from build123d import *

# Parameters (mm, degrees)
BOSS_EXTRU_1_DEPTH      = 1.5
BOSS_EXTRU_2_DEPTH      = 13.5
D_GAGEMENT_M32_D        = 3.4
D_GAGEMENT_M32_DEPTH    = 10
D_GAGEMENT_M32_TIP      = 1.021463052
D_GAGEMENT_M31_D        = 3.4
D_GAGEMENT_M31_DEPTH    = 10
D_GAGEMENT_M31_TIP      = 1.021463052
ESQUISSE12_W            = 13.5
ESQUISSE12_H            = 13.5
ENL_V_MAT_EXTRU_1_DEPTH = 1.5
CONG_1_R                = 1
CONG_2_R                = 1
D_GAGEMENT_M33_D        = 3.4
D_GAGEMENT_M33_DEPTH    = 10
D_GAGEMENT_M33_TIP      = 1.021463052


# Some blends are built 0.0001 mm under size
with BuildPart() as part:
    # Esquisse2 → Boss.-Extru.1 (new body)
    with BuildSketch(Plane.XY.offset(1.5)):
        Polygon((-25.392437762, 124.305889048), (-178.410591433, 124.305889048), (-178.410591433, 149.305889048), (-222.374284091, 149.305889048), (-222.374284091, 124.305889048), (-375.392437762, 124.305889048), (-375.392437762, 109.305889048), (-207.374284091, 109.305889048), (-207.374284091, 134.305889048), (-193.410591433, 134.305889048), (-193.410591433, 109.305889048), (-25.392437762, 109.305889048), align=None)
    extrude(amount=BOSS_EXTRU_1_DEPTH)

    # Esquisse3 → Boss.-Extru.2 (add)
    with BuildSketch(Plane.XY.offset(3)):
        Polygon((-375.392437762, 122.805889048), (-220.874284091, 122.805889048), (-220.874284091, 147.805889048), (-179.910591433, 147.805889048), (-179.910591433, 122.805889048), (-25.392437762, 122.805889048), (-25.392437762, 124.305889048), (-178.410591433, 124.305889048), (-178.410591433, 149.305889048), (-222.374284091, 149.305889048), (-222.374284091, 124.305889048), (-375.392437762, 124.305889048), align=None)
    extrude(amount=BOSS_EXTRU_2_DEPTH)

    # Dégagement M32
    with Locations(Plane(origin=(-229.874284091, 116.805889048, 3), x_dir=(1, 0, 0), z_dir=(0, 0, 1))):
        with Locations((0, 0), (-70.518153671, 0), (-138.018153671, 0), (58.963692658, 0), (129.481846329, 0), (196.981846329, 0)):
            Hole(D_GAGEMENT_M32_D / 2, depth=D_GAGEMENT_M32_DEPTH)
            with Locations((0, 0, -(D_GAGEMENT_M32_DEPTH + D_GAGEMENT_M32_TIP / 2))):  # 118° drill point
                Cone(0, D_GAGEMENT_M32_D / 2, D_GAGEMENT_M32_TIP, mode=Mode.SUBTRACT)

    # Dégagement M31
    with Locations(Plane(origin=(-214.874284091, 137.305889048, 3), x_dir=(1, 0, 0), z_dir=(0, 0, 1))):
        with Locations((0, 0), (28.963692658, 0)):
            Hole(D_GAGEMENT_M31_D / 2, depth=D_GAGEMENT_M31_DEPTH)
            with Locations((0, 0, -(D_GAGEMENT_M31_DEPTH + D_GAGEMENT_M31_TIP / 2))):  # 118° drill point
                Cone(0, D_GAGEMENT_M31_D / 2, D_GAGEMENT_M31_TIP, mode=Mode.SUBTRACT)

    # Esquisse12 → Enlèv. mat.-Extru.1 (cut)
    with BuildSketch(Plane.XY.offset(3)):
        with Locations((-214.124284091, 116.055889048)):
            Rectangle(ESQUISSE12_W, ESQUISSE12_H)
        with Locations((-186.660591433, 116.055889048)):
            Rectangle(ESQUISSE12_W, ESQUISSE12_H)
    extrude(amount=-ENL_V_MAT_EXTRU_1_DEPTH, mode=Mode.SUBTRACT)

    # Congé1
    # the kernel refuses this fillet: 1 mm, written as the material it adds along each edge
    with BuildSketch(Plane(origin=(-179.910591433, 122.805889048, 3), x_dir=(0, -1, 0), z_dir=(1, 0, 0))) as cong_1_piece_1:
        with BuildLine():
            CenterArc((CONG_1_R, -CONG_1_R), CONG_1_R, 90, 90)
            Line((0, -CONG_1_R), (0, 0))
            Line((0, 0), (CONG_1_R, 0))
        make_face()
    extrude(amount=154.518153671)
    with BuildSketch(Plane(origin=(-223.374284091, 147.805889048, 3), x_dir=(0, 0, 1), z_dir=(1, 0, 0))) as cong_1_piece_2_section:
        with BuildLine():
            CenterArc((CONG_1_R, CONG_1_R), CONG_1_R, 180, 90)
            Line((0, CONG_1_R), (0, 0))
            Line((0, 0), (CONG_1_R, 0))
        make_face()
    cong_1_piece_2 = extrude(amount=43.463692658, mode=Mode.PRIVATE)
    cong_1_piece_2 = split(cong_1_piece_2, bisect_by=Plane(origin=(-222.374284091, 147.582521109, 3.223367939), z_dir=(1, 0, 0)), keep=Keep.TOP, mode=Mode.PRIVATE)
    add(cong_1_piece_2)
    with BuildSketch(Plane(origin=(-375.392437762, 122.805889048, 3), x_dir=(0, 0, 1), z_dir=(1, 0, 0))) as cong_1_piece_3:
        with BuildLine():
            CenterArc((CONG_1_R, CONG_1_R), CONG_1_R, 180, 90)
            Line((0, CONG_1_R), (0, 0))
            Line((0, 0), (CONG_1_R, 0))
        make_face()
    extrude(amount=154.518153671)

    # Congé2
    cong_2_edges = [part.edges().sort_by_distance(p)[0] for p in [
        (-179.910591433, 134.805889048, 3),
        (-179.910591433, 147.512995829, 3.292893219),
        (-220.874284091, 147.512995829, 3.292893219),
        (-220.874284091, 134.805889048, 3),
        (-220.874284091, 147.805889048, 10.25),
        (-179.910591433, 147.805889048, 10.25),
    ]]
    fillet(cong_2_edges, radius=CONG_2_R - 0.0001)  # a hair under: the kernel refuses the full size

    # Dégagement M33
    with Locations(Plane(origin=(-92.892437762, 124.305889048, 9), x_dir=(1, 0, 0), z_dir=(0, 1, 0))):
        with Locations((0, 0), (52.5, -0.151530772), (-67.5, 0), (-147.5, 0), (-215, 0), (-267.5, 0)):
            Hole(D_GAGEMENT_M33_D / 2, depth=D_GAGEMENT_M33_DEPTH)
            with Locations((0, 0, -(D_GAGEMENT_M33_DEPTH + D_GAGEMENT_M33_TIP / 2))):  # 118° drill point
                Cone(0, D_GAGEMENT_M33_D / 2, D_GAGEMENT_M33_TIP, mode=Mode.SUBTRACT)


solid = part.part
Source: CAD feature listing. Evaluate the final solid. Frame: model axes, mm. A direction names the side the tool comes from. Give positions to 0.01 mm unless a question says otherwise; leave off trailing zeros. Write each loop counter-clockwise with the first axis right and the second up, starting at its lowest first coordinate (ties: lowest second). Pieces come first, ordered by that corner, then holes. Notation, with made-up numbers: M 53,21.5 L 109,21.5 A34 cw 109,51.5 Z; hole C -11,-21.5 d10. An arc over 180 degrees is marked long. Answer as a JSON object with one key per item and string values.
Q1. Cut plane A-A, the plane x = -323.5. Return the cut outline in (y, z), then the cut area to 3 significant figures.
Geometry check:
{"outline": "M 109.31,1.5 L 124.31,1.5 L 124.31,16.5 L 122.81,16.5 L 122.81,4 A1 cw 121.81,3 L 109.31,3 Z", "area": "43.0 mm^2"}
Q2. Contact query for flat-ended pins moving along their axis: P1, Ø2.5, axis at x = -215, z = 2.5, coming from the -Y side; P2, Ø1.2, axis at x = -197, z = 2.5, coming from the -Y side; P3, Ø4, axis at x = -265.5, z = 12, coming from the +Y side. Output: stop coordinate, or through.
Geometry check:
{"P1": "stops at y = 122.81", "P2": "stops at y = 134.31", "P3": "stops at y = 124.31"}
Q3. Access query for faces 1 (the face through (-200, 149.306, 9)), 2 (the face through (-220.874, 132, 9)), 3 (the face through (-101, 124.306, 9)), 4 (the face through (-214, 128, 1.5)), 5 (the face through (-104, 122.806, 10)). Directions: +Z, -Z, +X, -X, +Y, -Y. A direction counts if a zero-diameter tool reaches every point of the face in a straight line with its end or side. Return the directions, or none.
Geometry check:
{"face 1": "+Z, -Z, +X, -X, +Y", "face 2": "+Z, -Y", "face 3": "+Z, -Z, +X, +Y", "face 4": "-Z, +X, -X, +Y, -Y", "face 5": "+Z, +X, -X, -Y"}
Q4. Mould query, pull axis X, two halves, no side actions, for faces 6 (the face through (-298, 124.306, 9)), 7 (the face through (-222.374, 137, 9)), 8 (the face through (-179.911, 132, 11)). Classes: +X half, -X half, draft (parallel to the pull), parting line (faces both ways), or undercut.
Geometry check:
{"face 6": "draft", "face 7": "-X half", "face 8": "undercut"}
Q5. Ray query, line 1 along X through (y, z) = (141, 6.5); line 2 along X through (y, z) = (123, 7); line 3 along Y through (x, z) = (-317, 9.75). Return the intervals inside material, ascending.
Geometry check:
{"line 1": "x = -222.37 to -220.87, -179.91 to -178.41", "line 2": "x = -375.39 to -220.87, -179.91 to -25.39", "line 3": "y = 122.81 to 124.31"}
